from build123d import *

# Parameters (mm, degrees)
F0_W         = 69.85
F0_H         = 114.3
F0_R         = 2.3876
F0_W_2       = 9.525
F0_H_2       = 25.4
F1_DEPTH     = 5.08
F2_SIZE      = 5.07999
F4_DEPTH     = 2.54
F5_T1_DEPTH  = 71.5966436916
F5_T3_DEPTH  = 71.1214770669
F5_T8_DEPTH  = 29.3324993846
F5_T14_DEPTH = 29.5628780991
F6_R         = 1.27


# Not quite as in the source:
# - a fillet or chamfer that OpenCascade refuses, or shapes differently, is made with other operations: its cross-section is extruded or revolved along the edge and cut away or added
# - a fillet or chamfer is up to 0.001 mm smaller than in the source, because OpenCascade refuses the exact size


with BuildPart() as f1:
    # F0 (on Front) → F1 (new body)
    with BuildSketch(Plane.XZ):
        Rectangle(F0_W, F0_H)
        with Locations((0, -30.1625)):
            Circle(F0_R, mode=Mode.SUBTRACT)
        Rectangle(F0_W_2, F0_H_2, mode=Mode.SUBTRACT)
        with Locations((0, 30.1625)):
            Circle(F0_R, mode=Mode.SUBTRACT)
    extrude(amount=F1_DEPTH)

    # F2 (size 5.08 in the source; OpenCascade refuses exactly that, so slightly less here)
    f2_edges = [f1.edges().sort_by_distance(p)[0] for p in [
        (0, -5.08, 57.15),
        (34.925, -5.08, 0),
        (0, -5.08, -57.15),
        (-34.925, -5.08, 0),
    ]]
    chamfer(f2_edges, length=F2_SIZE)

    # F3 (on face) → F4 (join)
    with BuildSketch(Plane.XZ.offset(5.08)):
        with BuildLine():
            Line((10.4210752899, 45.360866621), (-9.7815324138, 45.7814973))
            Line((-9.7815324138, 45.7814973), (-23.4081424498, -1.9095465541))
            Line((-23.4081424498, -1.9095465541), (-19.9071371743, -18.2295814157))
            Line((-19.9071371743, -18.2295814157), (-4.5221770743, -23.345419034))
            Line((-4.5221770743, -23.345419034), (-12.6387388145, -10.1591296217))
            ThreePointArc((-12.6387388145, -10.1591296217), (-13.8432881685, -6.7829644544), (-13.5732137506, -3.2085427961))
            Line((-13.5732137506, -3.2085427961), (0, 43.2110093534))
            Line((0, 43.2110093534), (13.8653954743, -3.0792306258))
            ThreePointArc((13.8653954743, -3.0792306258), (14.1574638309, -6.6629312481), (12.9648391888, -10.0549602188))
            Line((12.9648391888, -10.0549602188), (4.856493974, -23.345419034))
            Line((4.856493974, -23.345419034), (20.4867540311, -18.2295814157))
            Line((20.4867540311, -18.2295814157), (23.789614439, -1.9095465541))
            Line((23.789614439, -1.9095465541), (10.4210752899, 45.360866621))
        make_face()
        Polygon((6.5450641223, -26.6576724823), (0, -23.345419034), (-6.802264601, -26.6576724823), (-27.4259783328, -18.2295814157), (-6.802264601, -32.0519991219), (0, -25.3795739263), (6.5450641223, -32.0519991219), (26.8477257341, -18.2295814157), align=None)
    extrude(amount=F4_DEPTH)

    # F5: fillet of radius 5.08 on 4 edges, made by hand

    # F5_s2 → F5_t1 (cut)
    with BuildSketch(Plane(origin=(14.3770362631, 0, 50.317420481), x_dir=(0, 1, 0), z_dir=(-0.2747322653, 0, -0.9615207655))):
        with BuildLine():
            ThreePointArc((-5.08, -21.9828009958), (-6.9394090512, -20.1233919446), (-7.62, -17.5833919446))
            Line((-7.62, -17.5833919446), (-7.62, -21.9828009958))
            Line((-7.62, -21.9828009958), (-5.08, -21.9828009958))
        make_face()
    extrude(amount=F5_T1_DEPTH, mode=Mode.SUBTRACT)

    # F5_s4 → F5_t3 (cut)
    with BuildSketch(Plane(origin=(5.2549558521, 0, -18.5812325171), x_dir=(0, 1, 0), z_dir=(-0.27213626, 0, 0.9622587261))):
        with BuildLine():
            ThreePointArc((-5.08, -22.3721072272), (-6.9394090512, -20.5126981759), (-7.62, -17.9726981759))
            Line((-7.62, -17.9726981759), (-7.62, -22.3721072272))
            Line((-7.62, -22.3721072272), (-5.08, -22.3721072272))
        make_face()
    extrude(amount=F5_T3_DEPTH, mode=Mode.SUBTRACT)


with BuildPart() as f5_tool6:
    # F5_s7 → F5_t8 (new body)
    with BuildSketch(Plane(origin=(25.7640738936, 0, -13.0383967217), x_dir=(0, 1, 0), z_dir=(-0.8922507056, 0, 0.4515403396))):
        with BuildLine():
            ThreePointArc((-5.08, 20.8299666066), (-6.9394090512, 22.6893756578), (-7.62, 25.2293756578))
            Line((-7.62, 25.2293756578), (-7.62, 20.8299666066))
            Line((-7.62, 20.8299666066), (-5.08, 20.8299666066))
        make_face()
    extrude(amount=F5_T8_DEPTH)

    split(bisect_by=Plane(origin=(10.401612722, 0, -25.0567324961), x_dir=(0, 1, 0), z_dir=(-0.3833998348, 0, 0.9235824634)), keep=Keep.TOP)

    split(bisect_by=Plane(origin=(9.1889369632, 0, -18.8710138282), x_dir=(0, 1, 0), z_dir=(0.4377909897, 0, -0.8990767761)), keep=Keep.TOP)


with BuildPart() as f1_1:
    add(f1.part)

    # F5_t5: cut F5_tool6
    add(f5_tool6.part, mode=Mode.SUBTRACT)


with BuildPart() as f5_tool12:
    # F5_s13 → F5_t14 (new body)
    with BuildSketch(Plane(origin=(0.6995793032, 0, 0.3406489008), x_dir=(0, 1, 0), z_dir=(-0.8990767761, 0, -0.4377909897))):
        with BuildLine():
            ThreePointArc((-5.08, 20.9893240819), (-6.9394090512, 22.8487331332), (-7.62, 25.3887331332))
            Line((-7.62, 25.3887331332), (-7.62, 20.9893240819))
            Line((-7.62, 20.9893240819), (-5.08, 20.9893240819))
        make_face()
    extrude(amount=F5_T14_DEPTH)

    split(bisect_by=Plane(origin=(-9.4055701954, 0, -18.5855524032), x_dir=(0, 1, 0), z_dir=(-0.4515403396, 0, -0.8922507056)), keep=Keep.TOP)

    split(bisect_by=Plane(origin=(-10.3083950149, 0, -25.2248565112), x_dir=(0, 1, 0), z_dir=(0.3782912807, 0, 0.9256866138)), keep=Keep.TOP)


with BuildPart() as f1_2:
    add(f1_1.part)

    # F5_t11: cut F5_tool12
    add(f5_tool12.part, mode=Mode.SUBTRACT)

    # F6
    f6_edges = [f1_2.edges().sort_by_distance(p)[0] for p in [
        (-2.3876, -5.08, 30.1625),
        (-2.3876, -5.08, -30.1625),
    ]]
    fillet(f6_edges, radius=F6_R)


solid = f1_2.part
Source: CAD feature listing. Evaluate the final solid. Frame: model axes, mm. A direction names the side the tool comes from. Round coordinates to 2 decimals unless told otherwise and drop trailing zeros. Answer as a JSON object with one key per item and string values. Group by question number.
Q1. Access query for faces 1 (the cylindrical face through (14.164, -6.332, -6.613)), 2 (the flat face through (-0.49, -2.58, -54.57)), 3 (the flat face through (-3.449, -6.332, -28.762)), 4 (the flat face through (12, -7.62, -26)), 5 (the flat face through (0, -3, 12.7)). Directions: +Z, -Z, +X, -X, +Y, -Y. A direction counts if a zero-diameter tool reaches every point of the face in a straight line with its end or side. Return the directions, or none.
Q2. Ray query, line 1 (Z direction, x = 0, y = -2.75); line 2 (Z direction, x = 0, y = -1.35); line 3 (Y direction, x = -24.5, z = 31). Return the intervals inside material, ascending. Write a range as from..to.
Q3. Section query A-A (y = -2.5). State how many separate pieces and enclosed holes the cut face has, plus the area to 3 significant figures.
Q4. Mould query, pull axis Z, two halves, no side actions, for faces 6 (the flat face through (-17.258, -6.332, -25.044)), 7 (the flat face through (0, -3, -12.7)), 8 (the flat face through (-0.49, -2.58, 54.57)). Classes: pulls with the +Z half, pulls with the -Z half, needs draft (parallel to the pull), parting line crosses it, or undercut.
Q5. Contact query for flat-ended pins moving along their axis: P1, Ø2.5, axis at x = -2, y = -2, coming from the -Z side; P2, Ø1.5, axis at y = -4, z = -3, coming from the +X side (3 decimals); P3, Ø4, axis at x = 24, z = -18.5, coming from the +Y side; P4, Ø2, axis at y = -4.5, z = -33.5, coming from the +X side (3 decimals). Output: stop coordinate, or through.
Completed:
{
 "1": {"face 1": "-Y", "face 2": "-Z, +X, -X, -Y", "face 3": "-Z, -Y", "face 4": "+Z, -Z, +X, -X, -Y", "face 5": "+Y, -Y"},
 "2": {"line 1": "-54.4..-32.55, -27.77..-12.7, 12.7..27.77, 32.55..54.4", "line 2": "-55.8..-32.55, -27.77..-12.7, 12.7..27.77, 32.55..55.8", "line 3": "-5.08..0"},
 "3": {"separate pieces": "1", "enclosed holes": "3", "area": "6,810 mm²"},
 "4": {"face 6": "pulls with the -Z half", "face 7": "undercut", "face 8": "pulls with the +Z half"},
 "5": {"P1": "z = -56.4", "P2": "x = 31.675", "P3": "y = 0", "P4": "x = 31.425"}
}
